For this review, take the finished solid that the model builds, in its own axes (mm). A direction names the side the tool comes from. Coordinates: 2 decimals unless noted, no trailing zeros. Write each loop counter-clockwise with the first axis right and the second up, starting at its lowest first coordinate (ties: lowest second). Pieces come first, ordered by that corner, then holes. Notation, with made-up numbers: (33.5, -19.5) - (42.5, -19.5) arc R27 cw to (42.5, 9.5) - close; hole circle Ø7 at (81, 31). An arc over 180 degrees is marked (long way). Write each question's results on one line, items separated by ' | '.
from build123d import *

# Parameters (mm, degrees)
SKETCH1_W           = 250.444
SKETCH1_H           = 134.366
SKETCH1_R           = 7.62
SKETCH1_R_2         = 2.794
SKETCH1_W_2         = 44.45
SKETCH1_H_2         = 25.4
BOSS_EXTRUDE1_DEPTH = 4.7625


with BuildPart() as part:
    # Sketch1 → Boss-Extrude1 (new body)
    with BuildSketch(Plane(origin=(0, 0, 0), x_dir=(1, 0, 0), z_dir=(0, 1, 0))):
        with Locations((-27.178, -17.907)):
            Rectangle(SKETCH1_W, SKETCH1_H)
        with Locations(Location((-50.8, 0, 0), (0, 0, 90))):
            Circle(SKETCH1_R, mode=Mode.SUBTRACT)
        with Locations(Location((-31.75, 0, 0), (0, 0, 90))):
            Circle(SKETCH1_R, mode=Mode.SUBTRACT)
        with Locations(Location((31.75, 0, 0), (0, 0, 90))):
            Circle(SKETCH1_R, mode=Mode.SUBTRACT)
        with Locations(Location((50.8, 0, 0), (0, 0, 90))):
            Circle(SKETCH1_R, mode=Mode.SUBTRACT)
        with Locations(Location((-139.7, 39.2684, 0), (0, 0, 90))):
            Circle(SKETCH1_R_2, mode=Mode.SUBTRACT)
        with Locations(Location((85.344, 39.2684, 0), (0, 0, 90))):
            Circle(SKETCH1_R_2, mode=Mode.SUBTRACT)
        with Locations(Location((88.0364, -18.034, 0), (0, 0, 90))):
            Circle(SKETCH1_R_2, mode=Mode.SUBTRACT)
        with Locations(Location((85.344, -75.0824, 0), (0, 0, 90))):
            Circle(SKETCH1_R_2, mode=Mode.SUBTRACT)
        with Locations(Location((-139.7, -75.0824, 0), (0, 0, 90))):
            Circle(SKETCH1_R_2, mode=Mode.SUBTRACT)
        with Locations(Location((-142.3924, -18.034, 0), (0, 0, 90))):
            Circle(SKETCH1_R_2, mode=Mode.SUBTRACT)
        Rectangle(SKETCH1_W_2, SKETCH1_H_2, mode=Mode.SUBTRACT)
    extrude(amount=BOSS_EXTRUDE1_DEPTH)


solid = part.part
Q1. Take a section at B-B on z = 0. State the section outline as (x, y) points (1 decimal), plus the area to 3 significant figures.
Results found:
outline: (-152.4, 0) - (-58.4, 0) - (-58.4, 4.8) - (-152.4, 4.8) - close; (-43.2, 0) - (-39.4, 0) - (-39.4, 4.8) - (-43.2, 4.8) - close; (-24.1, 0) - (-22.2, 0) - (-22.2, 4.8) - (-24.1, 4.8) - close; (22.2, 0) - (24.1, 0) - (24.1, 4.8) - (22.2, 4.8) - close; (39.4, 0) - (43.2, 0) - (43.2, 4.8) - (39.4, 4.8) - close; (58.4, 0) - (98, 0) - (98, 4.8) - (58.4, 4.8) - close | area: 691 mm2
Q2. For pin 1 (4.5 mm diameter, centred on x = 85.34, z = 75.08, fed in from -Y), flat-tipped, find the tip position at first contact; note if it passes through.
Results found:
pin 1: through
Q3. For faces 5 (the face through (-29, 4.762, 17)), 6 (the face through (0, 2, -12.7)), list the 3-axis set-ups (+Z, -Z, +X, -X, +Y, -Y) from which the entire face can be reached by the end or side of a thin tool; tool diameter is ignored.
Results found:
face 5: +Z, -Z, +X, -X, +Y | face 6: +Y, -Y
Q4. Mouldability with a two-part tool opening along X and no side actions: class faces 1 (the face through (98.044, 2, 19)), 2 (the face through (-29, 2, 85.09)), 3 (the face through (58.24, 2.35, 1.65)), 4 (the face through (-152.4, 2, 19)) as pulls with the +X half, pulls with the -X half, needs draft (parallel to the pull), parting line crosses it, or undercut.
Results found:
face 1: pulls with the +X half | face 2: needs draft | face 3: undercut | face 4: pulls with the -X half
Q5. Wall thickness on line 1 along X through (y, z) = (1.7, 75); line 2 along Z through (x, y) = (-2, 2.85); line 3 along Z through (x, y) = (-31.75, 2.9): over which ranges is each line inside the solid? List them lowest first. Write a range as from..to.
Results found:
line 1: -152.4..-142.49, -136.91..82.55, 88.14..98.04 | line 2: -49.28..-12.7, 12.7..85.09 | line 3: -49.28..-7.62, 7.62..85.09
Q6. Take a section at C-C on y = 3.15. State how many separate pieces and enclosed holes the cut face has, plus the area to 3 significant figures.
Results found:
separate pieces: 1 | enclosed holes: 11 | area: 31,600 mm2
Q7. Take a section at A-A on x = -50.8. State the section outline as (y, z) points.
Results found:
outline: (0, -49.28) - (4.76, -49.28) - (4.76, -7.62) - (0, -7.62) - close; (0, 7.62) - (4.76, 7.62) - (4.76, 85.09) - (0, 85.09) - close
